Can you work these out from the model? Positions are in its coordinate system, mm. A direction names the side the tool comes from. Round coordinates to 2 decimals unless told otherwise and drop trailing zeros. Order: outer loops, then holes, each group sorted by start corner. A loop starts at its lowest first (then second) coordinate and runs counter-clockwise, first axis right, second up. Notation, with made-up numbers: M 38.25,10 L 97.25,10 A24 cw 97.25,25 Z; hole C 54.5,51.25 d11. An arc over 180 degrees is marked long. Answer as a JSON object with one key per item and string values. Group by question number.
```python
from build123d import *

# Parameters (mm, degrees)
SKETCH_R        = 11
PAD_DEPTH       = 6.6
SKETCH001_R     = 11
SKETCH001_R_2   = 6
POCKET_DEPTH    = 4.3
SKETCH003_W     = 1.7
SKETCH003_H     = 1.7
PAD001_DEPTH    = 3
SKETCH004_W     = 2
SKETCH004_H     = 2
POCKET002_DEPTH = 4.3
SKETCH002_R     = 1.6
POCKET003_DEPTH = 6.601


with BuildPart() as part:
    # Sketch → Pad (new body)
    with BuildSketch(Plane.XY):
        Circle(SKETCH_R)
    extrude(amount=PAD_DEPTH)

    # Sketch001 → Pocket (cut)
    with BuildSketch(Plane(origin=(0, 0, 0), x_dir=(1, 0, 0), z_dir=(0, 0, -1))):
        Circle(SKETCH001_R)
        Circle(SKETCH001_R_2, mode=Mode.SUBTRACT)
    extrude(amount=-POCKET_DEPTH, mode=Mode.SUBTRACT)

    # Sketch003 → Pad001 (new body)
    with BuildSketch(Plane(origin=(0, 0, 0), x_dir=(1, 0, 0), z_dir=(0, 0, -1))):
        with Locations((0, 4.35)):
            Rectangle(SKETCH003_W, SKETCH003_H)
        with Locations((0, -4.35)):
            Rectangle(SKETCH003_W, SKETCH003_H)
    extrude(amount=PAD001_DEPTH)

    # Sketch004 → Pocket002 (cut)
    with BuildSketch(Plane(origin=(0, 0, 0), x_dir=(1, 0, 0), z_dir=(0, 0, -1))):
        with Locations((-4.2, 0)):
            Rectangle(SKETCH004_W, SKETCH004_H)
        with Locations((4.2, 0)):
            Rectangle(SKETCH004_W, SKETCH004_H)
    extrude(amount=-POCKET002_DEPTH, mode=Mode.SUBTRACT)

    # Sketch002 → Pocket003 (cut, through all)
    with BuildSketch(Plane(origin=(0, 0, 0), x_dir=(1, 0, 0), z_dir=(0, 0, -1))):
        Circle(SKETCH002_R)
    extrude(amount=-POCKET003_DEPTH, mode=Mode.SUBTRACT)


solid = part.part
```
1) If we section it at B-B on y = 0: Write out the boundary of the cut face in (x, z), plus the area to 3 significant figures.
2) If we section it at A-A on x = 0: Write out the boundary of the cut face in (y, z).
3) If we section it at D-D on y = 3: Write out the boundary of the cut face in (x, z), plus the area to 3 significant figures.
4) I need wall thicknesses on line 1 along X through (y, z) = (0, 4.25); line 2 along Y through (x, z) = (0, 4); line 3 along Z through (x, y) = (-6.5, -7.75). Which ranges of each line are inside material? Lowest first, please.
5) If we section it at C-C on z = -1.75: Write out the boundary of the cut face in (x, y), plus the area to 3 significant figures.
6) Which directions (+Z, -Z, +X, -X, +Y, -Y) give clear straight access to the entire face, cutting with the end or side of a thin tool? Please do faces 1 (the face through (0.85, -4, -1)), 2 (the face through (-0.85, -4, -1)), 3 (the face through (5.2, 0, 2)).
7) We'd pull the mould along Y, two halves only. Please class faces 4 (the face through (0, 5.2, -1)), 5 (the face through (-5.2, 0, 2)), 6 (the face through (5, 5, 4.3)), 7 (the face through (-4, -1, 2)): +Y half, -Y half, draft (parallel to the pull), parting line (faces both ways), or undercut.
8) For pin 1 (2 mm diameter, centred on y = 0, z = 2, fed in from +X); pin 2 (0.8 mm diameter, centred on y = 4, z = -1.5, fed in from +X); pin 3 (2 mm diameter, centred on x = -2, y = 2.5, fed in from -Z); pin 4 (1.5 mm diameter, centred on x = 8, z = 3.5, fed in from -Y), each with a flat end and sliding along its axis, tell me the tip position at first contact or that it passes through.
Findings:
{
 "1": {"outline": "M -11,4.3 L -6,4.3 L -6,0 L -5.2,0 L -5.2,4.3 L -3.2,4.3 L -3.2,0 L -1.6,0 L -1.6,6.6 L -11,6.6 Z; M 1.6,0 L 3.2,0 L 3.2,4.3 L 5.2,4.3 L 5.2,0 L 6,0 L 6,4.3 L 11,4.3 L 11,6.6 L 1.6,6.6 Z", "area": "63.9 mm^2"},
 "2": {"outline": "M -11,4.3 L -6,4.3 L -6,0 L -5.2,0 L -5.2,-3 L -3.5,-3 L -3.5,0 L -1.6,0 L -1.6,6.6 L -11,6.6 Z; M 1.6,0 L 3.5,0 L 3.5,-3 L 5.2,-3 L 5.2,0 L 6,0 L 6,4.3 L 11,4.3 L 11,6.6 L 1.6,6.6 Z"},
 "3": {"outline": "M -10.58,4.3 L -5.2,4.3 L -5.2,0 L 5.2,0 L 5.2,4.3 L 10.58,4.3 L 10.58,6.6 L -10.58,6.6 Z", "area": "93.4 mm^2"},
 "4": {"line 1": "x = -6 to -5.2, -3.2 to -1.6, 1.6 to 3.2, 5.2 to 6", "line 2": "y = -6 to -1.6, 1.6 to 6", "line 3": "z = 4.3 to 6.6"},
 "5": {"outline": "M -0.85,-5.2 L 0.85,-5.2 L 0.85,-3.5 L -0.85,-3.5 Z; M -0.85,3.5 L 0.85,3.5 L 0.85,5.2 L -0.85,5.2 Z", "area": "5.78 mm^2"},
 "6": {"face 1": "-Z, +X, +Y, -Y", "face 2": "-Z, -X, +Y, -Y", "face 3": "-Z"},
 "7": {"face 4": "+Y half", "face 5": "undercut", "face 6": "draft", "face 7": "undercut"},
 "8": {"pin 1": "stops at x = 6", "pin 2": "stops at x = 0.85", "pin 3": "stops at z = 0", "pin 4": "passes through"}
}
